```python
from build123d import *

# Parameters (mm, degrees)
SKETCH7_W          = 10
SKETCH7_H          = 1.5
CUT_EXTRUDE4_DEPTH = 1.5
SKETCH8_W          = 10
SKETCH8_H          = 1.7
CUT_EXTRUDE5_DEPTH = 1.5


with BuildPart() as part:
    # Sketch1 → Revolve1 (revolve)
    with BuildSketch(Plane(origin=(0, 0, 0), x_dir=(0, 0, -1), z_dir=(1, 0, 0)), mode=Mode.PRIVATE) as revolve1_sk:
        Polygon((-134.992104591, 0), (165.007895409, 0), (165.007895409, 4.5), (149.357384883, 4.5), (149.357384883, 5), (59.357384883, 5), (59.357384883, 6), (19.357384883, 6), (19.357384883, 5), (-134.992104591, 5), align=None)
    revolve(revolve1_sk.sketch.rotate(Axis((0, 0, 134.992104591), (0, 0, -1)), 90), axis=Axis((0, 0, 134.992104591), (0, 0, -1)))

    # Sketch7 → Cut-Extrude4 (cut, symmetric)
    with BuildSketch(Plane(origin=(0, 0, 0), x_dir=(0, 0, -1), z_dir=(1, 0, 0))):
        with Locations((51.512242661, 5.25)):
            Rectangle(SKETCH7_W, SKETCH7_H)
    extrude(amount=CUT_EXTRUDE4_DEPTH, both=True, mode=Mode.SUBTRACT)

    # Sketch8 → Cut-Extrude5 (cut, symmetric)
    with BuildSketch(Plane(origin=(0, 0, 0), x_dir=(0, 0, -1), z_dir=(1, 0, 0))):
        with Locations((156.934482796, 3.65)):
            Rectangle(SKETCH8_W, SKETCH8_H)
    extrude(amount=CUT_EXTRUDE5_DEPTH, both=True, mode=Mode.SUBTRACT)


solid = part.part
```
Could you check a few things on this model? Use its own coordinates, in mm. A direction names the side the tool comes from. Coordinates: 2 decimals unless noted, no trailing zeros. Write each loop counter-clockwise with the first axis right and the second up, starting at its lowest first coordinate (ties: lowest second). Pieces come first, ordered by that corner, then holes. Notation, with made-up numbers: (32, -8.5) -> (47, -8.5) arc R15 ccw to (47, 4.5) -> close; hole circle Ø8 at (89, -13). An arc over 180 degrees is marked (long way). Return JSON: item names as keys, results as strings.
(1) Which directions (+Z, -Z, +X, -X, +Y, -Y) give clear straight access to the entire face, cutting with the end or side of a thin tool? Please do faces 1 (the flat face through (0, 0, 134.992)), 2 (the cylindrical face through (-0.59, -4.46, -157.07)), 3 (the cylindrical face through (-5, 0, 59)).
Numbers:
{"face 1": "+Z, +X, -X, +Y, -Y", "face 2": "-Z", "face 3": "+Z"}
(2) Imagine slicing it at A-A, the plane y = 0. Please give me the cut outline in (x, z).
Numbers:
{"outline": "(-6, -59.36) -> (-5, -59.36) -> (-5, -149.36) -> (-4.5, -149.36) -> (-4.5, -165.01) -> (4.5, -165.01) -> (4.5, -149.36) -> (5, -149.36) -> (5, -59.36) -> (6, -59.36) -> (6, -19.36) -> (5, -19.36) -> (5, 134.99) -> (-5, 134.99) -> (-5, -19.36) -> (-6, -19.36) -> close"}
(3) I'm going to push flat-ended pins straight in: pin 1 (3 mm diameter, centred on x = 3, z = 63, fed in from -Y); pin 2 (3.5 mm diameter, centred on x = 0, z = -155, fed in from +Y); pin 3 (0.7 mm diameter, centred on y = 4, z = -157, fed in from -X); pin 4 (5 mm diameter, centred on x = 4, y = 3, fed in from -Z). Where does each tip first touch, or does it pass through?
Numbers:
{"pin 1": "stops at y = -4.77", "pin 2": "stops at y = 4.24", "pin 3": "stops at x = -2.63", "pin 4": "stops at z = -165.01"}
(4) Imagine slicing it at B-B, the plane z = -108. Please give me the cut outline in (x, y), then the cut area to 3 significant figures.
Numbers:
{"outline": "circle Ø10 at (0, 0)", "area": "78.5 mm2"}
(5) I need wall thicknesses on L1, parallel to X at y = 2.25, z = -82; L2, parallel to Z at x = 5, y = -1.25; L3, parallel to Y at x = -0.5, z = 45. Which ranges of each line are inside material? Lowest first, please.
Numbers:
{"L1": "x = -4.47 to 4.47", "L2": "z = -59.36 to -19.36", "L3": "y = -4.97 to 4.97"}
